Part model, mm, in its own coordinate system. Face numbers are marked on the shaded views. Round coordinates to 2 decimals unless told otherwise and drop trailing zeros. Loops run counter-clockwise (first coordinate to the right, second up) from the corner with the lowest first, then second, coordinate; pieces in that order, holes last.
(1) Cut at A-A on y = 158. List the corners of the cut face in (x, z).
(2) Probe probe 1 along Y at (x, z) = (159, -8); probe 2 along Y at (x, z) = (154.5, -32.5); probe 3 along X at (y, z) = (155.25, -16). List the from-to ranges inside material, lowest first.
(3) Mould opens along Y. For the marked faces 1 and 2 say: +Y half, -Y half, draft (parallel to the pull), parting line (faces both ways), or undercut.
(4) Cut at B-B on x = 160.5. List the corners of the cut face in (y, z), then the cut area to 3 significant figures.
(5) Flat gauge pins, fed straight in: pin 1 (1.5 mm diameter, centred on y = 162, z = -22, fed in from +X); pin 2 (1.5 mm diameter, centred on y = 161.5, z = -23, fed in from -X); pin 3 (1 mm diameter, centred on x = 154.5, z = 5, fed in from +Y). Where does each tip first touch, or does it go through?
(6) Cut at C-C on z = -45. List the corners of the cut face in (x, y) (3 decimals).
from build123d import *

# Parameters (mm, degrees)
EXTRUDE1_DEPTH          = 45
EXTRUDE1_DEPTH_BACK     = 56
SKETCH1_R               = 6
EXTRUDE2_DEPTH          = 41
EXTRUDE2_DEPTH_BACK     = 52.5
SKETCH2_R               = 6.35
CUT_EXTRUDE1_DEPTH      = 241.588362675
CUT_EXTRUDE1_DEPTH_BACK = 241.588362675
SKETCH3_R               = 4.365


with BuildPart() as part:
    # Sketch1 → Extrude1 (new, two sides: drawn at the far end of the back side and taken through both)
    with BuildSketch(Plane.XY.offset(-EXTRUDE1_DEPTH_BACK)):
        with Locations(Location((159.099025767, 159.099025767, 0), (0, 0, 180))):
            Circle(SKETCH1_R)
    extrude(amount=EXTRUDE1_DEPTH + EXTRUDE1_DEPTH_BACK)

    # Sketch2 → Extrude2 (add, two sides: drawn at the far end of the back side and taken through both)
    with BuildSketch(Plane.XY.offset(-EXTRUDE2_DEPTH_BACK)):
        with Locations(Location((159.099025767, 159.099025767, 0), (0, 0, 180))):
            Circle(SKETCH2_R)
    extrude(amount=EXTRUDE2_DEPTH + EXTRUDE2_DEPTH_BACK)

    # Sketch3 → Cut-Extrude1 (cut, two sides: drawn at the far end of the back side and taken through both)
    with BuildSketch(Plane.XY.offset(-CUT_EXTRUDE1_DEPTH_BACK)):
        with Locations((159.099025767, 159.099025767)):
            Circle(SKETCH3_R)
    extrude(amount=CUT_EXTRUDE1_DEPTH + CUT_EXTRUDE1_DEPTH_BACK, mode=Mode.SUBTRACT)


solid = part.part
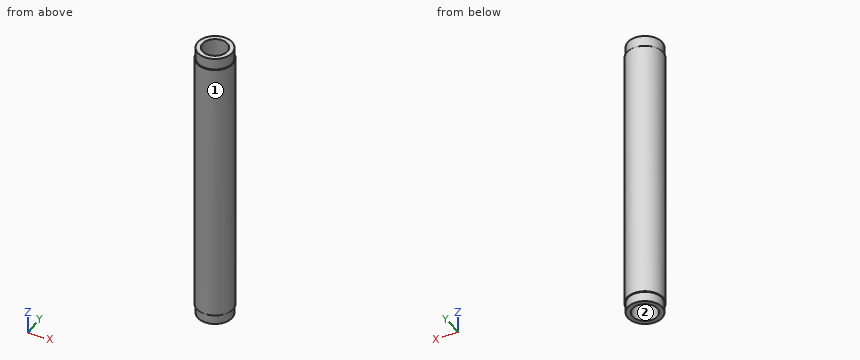
Final values:
1. outline: (152.84, -52.5) - (153.2, -52.5) - (153.2, -56) - (154.87, -56) - (154.87, 45) - (153.2, 45) - (153.2, 41) - (152.84, 41) - close; (163.32, -56) - (165, -56) - (165, -52.5) - (165.35, -52.5) - (165.35, 41) - (165, 41) - (165, 45) - (163.32, 45) - close
2. probe 1: y = 152.75 to 154.74, 163.46 to 165.45
2. probe 2: y = 154.72 to 163.48
2. probe 3: x = 154.05 to 157.04, 161.16 to 164.15
3. face 1: parting line
3. face 2: undercut
4. outline: (152.91, -52.5) - (153.26, -52.5) - (153.26, -56) - (154.96, -56) - (154.96, 45) - (153.26, 45) - (153.26, 41) - (152.91, 41) - close; (163.23, -56) - (164.93, -56) - (164.93, -52.5) - (165.29, -52.5) - (165.29, 41) - (164.93, 41) - (164.93, 45) - (163.23, 45) - close
4. area: 411 mm2
5. pin 1: stops at x = 165.07
5. pin 2: stops at x = 152.97
5. pin 3: stops at y = 163.95
6. outline: circle Ø12.7 at (159.099, 159.099); hole circle Ø8.73 at (159.099, 159.099)
